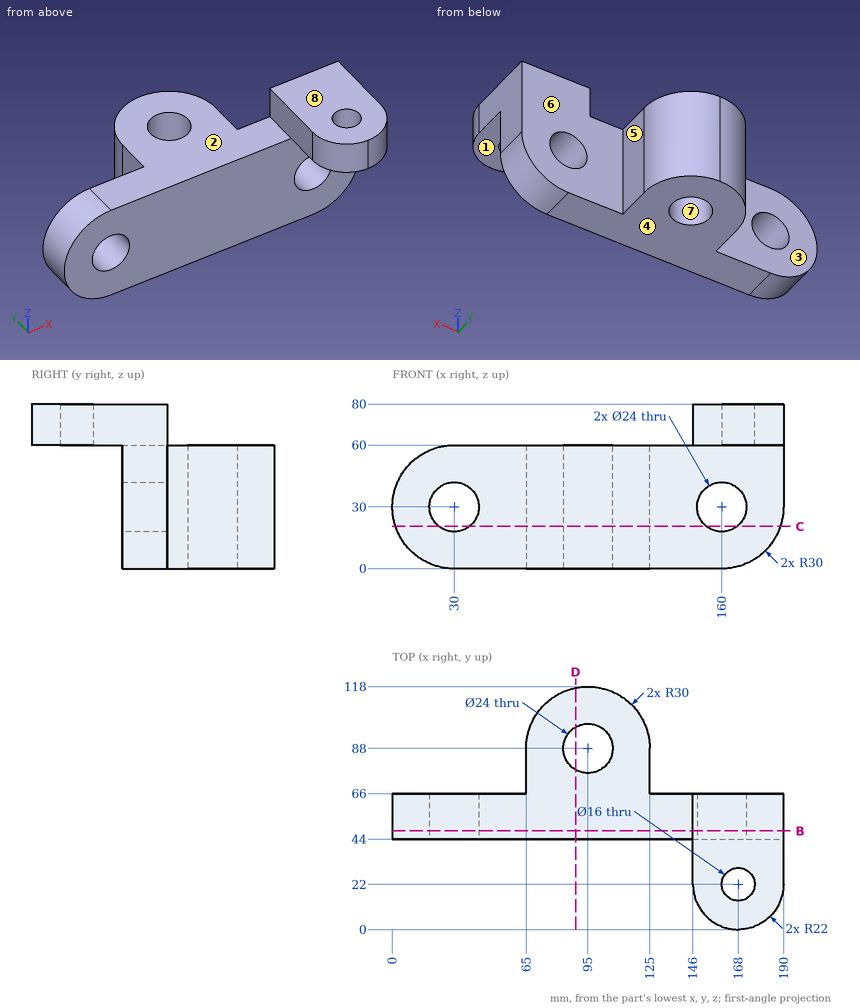
Design review of the part shown in the three views and the two pictorial views. Dimensions are in mm from the part's minimum x, y and z. A direction names the side the tool comes from. Coordinates: 2 decimals unless noted, no trailing zeros. Write each loop counter-clockwise with the first axis right and the second up, starting at its lowest first coordinate (ties: lowest second). Pieces come first, ordered by that corner, then holes. Notation, with made-up numbers: (10, 73) -> (36, 73) arc R22 ccw to (36, 100) -> close; hole circle Ø6 at (-29, -29.75). An arc over 180 degrees is marked (long way). Answer in a Markdown table with one row per item.
1. We need section C-C, the plane z = 20.5. Give the number of separate pieces and of enclosed holes in the cut face, and give its area (3 significant figures).
Answers below:
| item | result |
|---|---|
| separate pieces | 3 |
| enclosed holes | 1 |
| area | 5,750 mm^2 |
2. Wall thickness on probe 1 along X at (y, z) = (57, 30); probe 2 along X at (y, z) = (87.5, 53); probe 3 along Y at (x, z) = (95, 24): over which ranges is each line inside the solid? List them lowest first. Write a range as [from, to].
Answers below:
| item | result |
|---|---|
| probe 1 | x = [0, 18], [42, 148], [172, 190] |
| probe 2 | x = [65, 83.01], [106.99, 125] |
| probe 3 | y = [44, 76], [100, 118] |
3. Clearance check with flat-ended pins moving along their axes: pin 1 Ø16 at (y, z) = (47, 65.5) entering from -X; pin 2 Ø5 at (y, z) = (99.5, 50) entering from +X; pin 3 Ø14.5 at (x, z) = (160, 30) entering from -Y; pin 4 Ø1 at (x, z) = (40.5, 50) entering from -Y. State where each tip first meets the part, or that it passes through.
Answers below:
| item | result |
|---|---|
| pin 1 | stops at x = 18.01 |
| pin 2 | stops at x = 123.62 |
| pin 3 | passes through |
| pin 4 | stops at y = 44 |
4. We need section B-B, the plane y = 48. State the section outline as (x, z) points.
Answers below:
| item | result |
|---|---|
| outline | (30, 0) -> (160, 0) arc R30 ccw to (190, 30) -> (190, 80) -> (146, 80) -> (146, 60) -> (30, 60) arc R30 ccw to start; hole circle Ø24 at (30, 30); hole circle Ø24 at (160, 30) |
5. For the marked faces 1, 2, 3, 4 and 5, list the 3-axis set-ups (+Z, -Z, +X, -X, +Y, -Y) from which the entire face can be reached by the end or side of a thin tool; tool diameter is ignored.
Answers below:
| item | result |
|---|---|
| face 1 | -Z, +X, -X, -Y |
| face 2 | +Z, -X, +Y, -Y |
| face 3 | +Z, -Z, -X, +Y |
| face 4 | -Z, +X, -X, +Y, -Y |
| face 5 | +Z, -Z, +X, +Y |
6. We need section D-D, the plane x = 89. State the section outline as (y, z) points.
Answers below:
| item | result |
|---|---|
| outline | (44, 0) -> (77.61, 0) -> (77.61, 60) -> (44, 60) -> close; (98.39, 0) -> (117.39, 0) -> (117.39, 60) -> (98.39, 60) -> close |
7. Draft analysis for pull direction Y (two halves, no side actions). For the marked faces 6, 7 and 8, state which applies: +Y half, -Y half, draft (parallel to the pull), parting line (faces both ways), or undercut.
Answers below:
| item | result |
|---|---|
| face 6 | +Y half |
| face 7 | undercut |
| face 8 | draft |
